Verification items for this drawing (mm, ordinates from the low corner). A direction names the side the tool comes from. Give positions to 0.01 mm unless a question says otherwise; leave off trailing zeros. Order: outer loops, then holes, each group sorted by start corner. A loop starts at its lowest first (then second) coordinate and runs counter-clockwise, first axis right, second up. Notation, with made-up numbers: M 29,76.25 L 50,76.25 A16 ccw 50,94.25 Z; hole C 1,-22 d4. An arc over 180 degrees is marked long. Return JSON: item names as keys, results as strings. Group by question number.
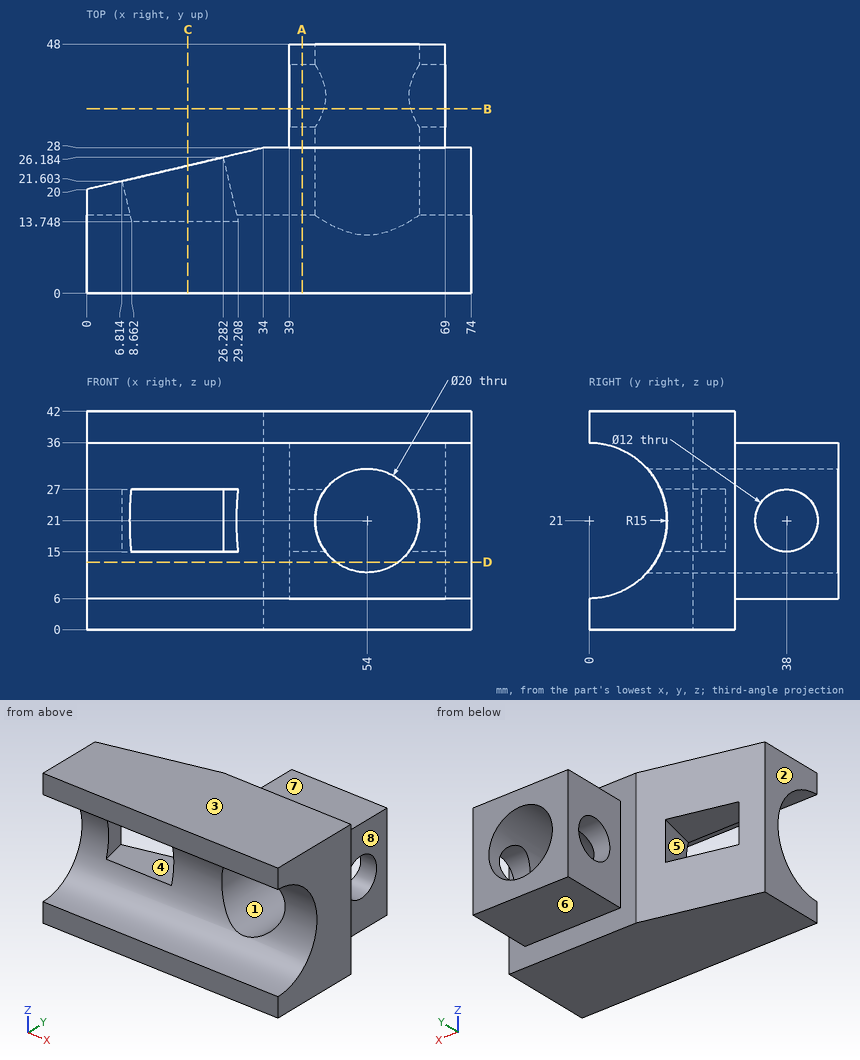
1) Sectioned sample at A-A on x = 41.5. Record the boundary of the cut face in (y, z).
2) Sectioned sample at B-B on y = 35.5. Record the boundary of the cut face in (x, z) (1 decimal).
3) Depth check by flat-ended pin: P1, Ø10, axis at y = 35, z = 20, coming from the -X side; P2, Ø10, axis at x = 54.5, y = 36, coming from the -Z side; P3, Ø6, axis at x = 48, y = 38, coming from the +Z side. Enter the tip coordinate at first touch or a pass-through.
4) Tool access check on the marked faces 5, 6, 7 and 8. Record the directions out of +Z, -Z, +X, -X, +Y, -Y that give a thin tool (end or side, any length) a straight path to the whole face; none if there is none.
5) Sectioned sample at D-D on z = 13. Record the boundary of the cut face in (x, y), then the cut area to 3 significant figures.
6) Sectioned sample at C-C on x = 19.5. Record the boundary of the cut face in (y, z), then the cut area to 3 significant figures.
7) Material ranges on line 1 along Z through (x, y) = (11.5, 21); line 2 along Y through (x, z) = (43, 21); line 3 along Y through (x, z) = (70.5, 11), recorded low to high.
8) Release check for a two-part mould opening along X. For the marked faces 1, 2, 3 and 4 record: released by +X, released by -X, zero draft, split by the parting line, or undercut.
Reply:
{
 "1": {"outline": "M 0,0 L 28,0 L 28,6 L 48,6 L 48,36 L 28,36 L 28,42 L 0,42 L 0,36 A15 cw 0,6 Z; hole C 38,21 d12"},
 "2": {"outline": "M 39,6 L 69,6 L 69,15.5 L 62.4,15.5 A10 cw 45.6,15.5 L 39,15.5 Z; M 39,26.5 L 45.6,26.5 A10 cw 62.4,26.5 L 69,26.5 L 69,36 L 39,36 Z"},
 "3": {"P1": "x = 39", "P2": "z = 6", "P3": "z = 36"},
 "4": {"face 5": "-Y", "face 6": "-Z, +X, -X, +Y", "face 7": "+Z, +X, -X, +Y", "face 8": "+Z, -Z, +X, +Y"},
 "5": {"outline": "M 0,12.69 L 48,12.69 L 48,48 L 39,48 L 39,28 L 34,28 L 0,20 Z; M 60,12.69 L 74,12.69 L 74,28 L 69,28 L 69,48 L 60,48 Z", "area": "1,170 mm^2"},
 "6": {"outline": "M 0,0 L 24.59,0 L 24.59,15 L 13.75,15 A15 cw 0,6 Z; M 0,36 A15 cw 13.75,27 L 24.59,27 L 24.59,42 L 0,42 Z", "area": "559 mm^2"},
 "7": {"line 1": "0 to 15, 27 to 42", "line 2": "15 to 32, 44 to 48", "line 3": "11.18 to 28"},
 "8": {"face 1": "undercut", "face 2": "released by -X", "face 3": "zero draft", "face 4": "undercut"}
}
